Input: part model. Units: mm. Frame: model coordinates. A direction names the side the tool comes from. Give positions to 0.01 mm unless a question says otherwise; leave off trailing zeros. Order: outer loops, then holes, each group sorted by start corner. A loop starts at its lowest first (then second) coordinate and runs counter-clockwise, first axis right, second up. Notation, with made-up numbers: (17.25, -19) - (39.25, -19) arc R23 ccw to (39.25, 5) - close; hole circle Ø4 at (81.5, 10.5). An arc over 180 degrees is marked (long way). Answer in a Markdown table with one row per item. Add a question column.
1. Section query B-B on x = 50. Return loops of the section in (y, z) (1 decimal), and give its area (3 significant figures).
2. Access query for faces 5 (the face through (-4, 50.8, -23)), 6 (the face through (280.988, 3, -15)). Directions: +Z, -Z, +X, -X, +Y, -Y. A direction counts if a zero-diameter tool reaches every point of the face in a straight line with its end or side. Return the directions, or none.
3. Ray query, line 1 (Y direction, x = 109.5, z = 36) (3 decimals); line 2 (Y direction, x = -187.5, z = -9.5) (3 decimals); line 3 (Z direction, x = 96, y = 49.5). Return the intervals inside material, ascending. Write a range as [from, to].
4. Section query C-C on z = 41. Return loops of the section in (x, y) (1 decimal), and give its area (3 significant figures).
5. Section query D-D on y = 15. Return loops of the section in (x, z), and give its area (3 significant figures).
6. Mould query, pull axis Y, two halves, no side actions, for faces 1 (the face through (5, 3.175, 2)), 2 (the face through (4, 0, 1)), 3 (the face through (-277.812, 29, 2)), 4 (the face through (217.632, 52.41, 5.074)). Classes: released by +Y, released by -Y, zero draft, split by the parting line, or undercut.
7. Contact query for flat-ended pins moving along their axis: pin 1 (2 mm diameter, centred on y = 10, z = 14, fed in from +X); pin 2 (3.5 mm diameter, centred on y = 52, z = -0.5, fed in from +X); pin 3 (8 mm diameter, centred on x = -93, y = 13.5, fed in from +Z). Output: stop coordinate, or through.
8. Section query A-A on z = -32. Return loops of the section in (x, y) (1 decimal), and give its area (3 significant figures).
Autodesk Inventor part; units mm, degrees
ref_plane "YZ Plane" through (0, 0, 0) normal (1, 0, 0) x (0, 1, 0)
ref_plane "XZ Plane" through (0, 0, 0) normal (0, 1, 0) x (-1, 0, 0)
ref_plane "XY Plane" through (0, 0, 0) normal (0, 0, 1) x (1, 0, 0)
sketch "Sketch1" plane through (0, 0, 0) normal (0, 1, 0) x (-1, 0, 0)
  line L0 (-280.9875, -52.3875) -> (-280.9875, 52.3875)
  line L1 (-280.9875, 52.3875) -> (280.9875, 52.3875)
  line L2 (280.9875, 52.3875) -> (280.9875, -52.3875)
  line L3 (280.9875, -52.3875) -> (-280.9875, -52.3875)
  line L4 (-280.9875, -52.3875) -> (280.9875, 52.3875) construction
  line L5 (-280.9875, 52.3875) -> (280.9875, -52.3875) construction
  line L6 (0, -52.3875) -> (0, -17.4625) construction
  line L7 (-277.8125, -49.2125) -> (277.8125, -49.2125)
  line L8 (277.8125, -49.2125) -> (277.8125, 49.2125)
  line L9 (277.8125, 49.2125) -> (-277.8125, 49.2125) construction
  line L10 (-277.8125, 49.2125) -> (-277.8125, -49.2125)
  line L11 (-277.8125, -49.2125) -> (277.8125, 49.2125) construction
  line L12 (277.8125, -49.2125) -> (-277.8125, 49.2125) construction
  line L13 (277.8125, 49.2125) -> (277.8125, 52.3875)
  line L14 (-277.8125, 49.2125) -> (-277.8125, 52.3875)
  point P0 (0, 0)
  dimension "d0" = 104.775
  dimension "d1" = 561.975
  dimension "d2" = 34.925
  dimension "d3" = 555.625
  dimension "d4" = 98.425
extrude "Extrusion1" add sketch "Sketch1" along normal blind 3.175 contours L1 L13 L8 L7 L10 L14
extrude "Extrusion2" add sketch "Sketch1" along normal blind 50.8 contours L0 L1 L14 L10 L7 L8 L13 L2 L3
sketch "Sketch2" plane through (0, 50.8, 0) normal (0, 1, 0) x (1, 0, 0)
  line L0 (-280.9875, -52.3875) -> (-277.8125, -52.3875)
  line L1 (-280.9875, -52.3875) -> (255.5875, -52.3875)
  line L2 (280.9875, -52.3875) -> (280.9875, -26.9875)
  line L3 (-280.9875, -26.9875) -> (-280.9875, -52.3875)
  line L4 (-280.9875, 52.3875) -> (-280.9875, -52.3875)
  line L5 (-280.9875, 52.3875) -> (255.5875, 52.3875)
  line L6 (280.9875, 52.3875) -> (280.9875, 17.4625)
  line L7 (-280.9875, 17.4625) -> (-280.9875, 52.3875)
  line L8 (-280.9875, 52.3875) -> (-255.5875, 52.3875)
  line L9 (-255.5875, -52.3875) -> (-280.9875, -52.3875)
  line L10 (-280.9875, -52.3875) -> (-280.9875, -26.9875)
  line L11 (-277.8125, -52.3875) -> (277.8125, -52.3875)
  line L12 (280.9875, 52.3875) -> (255.5875, 52.3875)
  line L13 (255.5875, -52.3875) -> (280.9875, -52.3875)
  line L14 (280.9875, -52.3875) -> (280.9875, 17.4625)
  line L15 (255.5875, 17.4625) -> (255.5875, -26.9875)
  line L16 (255.5875, 17.4625) -> (-255.5875, 17.4625)
  line L17 (255.5875, 52.3875) -> (280.9875, 52.3875)
  line L18 (280.9875, 17.4625) -> (280.9875, 52.3875)
  line L19 (255.5875, -26.9875) -> (-255.5875, -26.9875)
  line L20 (255.5875, -52.3875) -> (280.9875, -52.3875)
  line L21 (-255.5875, 17.4625) -> (-255.5875, -26.9875)
  line L22 (-280.9875, 17.4625) -> (-280.9875, 52.3875)
  line L23 (-280.9875, -26.9875) -> (-280.9875, 17.4625)
  line L24 (-277.8125, -52.3875) -> (-277.8125, 49.2125) construction
  line L25 (-277.8125, -52.3875) -> (-277.8125, -49.2125) construction
  line L26 (-277.8125, -49.2125) -> (277.8125, -49.2125)
  line L27 (-277.8125, -49.2125) -> (-277.8125, -52.3875)
  line L28 (277.8125, -49.2125) -> (277.8125, -52.3875)
  point P0 (0, 0)
  dimension "d9" = 561.975
  dimension "d10" = 25.4
  dimension "d11" = 561.975
  dimension "d12" = 34.925
  dimension "d13" = 25.4
  dimension "d14" = 104.775
  dimension "d15" = 25.4
  dimension "d18" = 3.175
  dimension "d19" = 555.625
extrude "Extrusion3" add sketch "Sketch2" along normal blind 3.175
sketch "Sketch3" plane through (0, 53.975, 0) normal (0, 1, 0) x (1, 0, 0)
  line L0 (-277.8125, -52.3875) -> (-277.8125, 49.2125)
  line L1 (-277.8125, -52.3875) -> (277.8125, -52.3875)
  line L2 (277.8125, -52.3875) -> (277.8125, -49.2125)
  line L3 (277.8125, -49.2125) -> (-277.8125, -49.2125)
  line L4 (-277.8125, -49.2125) -> (-277.8125, -52.3875)
  point P0 (0, 0)
  dimension "d20" = 555.625
  dimension "d21" = 3.175
extrude "Extrusion4" cut sketch "Sketch3" against normal blind 3.175
sketch "Sketch4" plane through (280.9875, 0, 52.3875) normal (1, 0, 0) x (0, 0, -1)
  line L0 (3.175, 53.975) -> (0, 53.975)
  line L1 (0, 53.975) -> (104.775, 53.975)
  line L2 (104.775, 53.975) -> (104.775, 0)
  line L3 (0, 0) -> (0, 53.975)
  line L4 (52.3875, 0) -> (52.3875, 3.175) construction
  line L5 (0, 3.175) -> (101.6, 3.175) construction
  line L6 (0, 3.175) -> (104.775, 3.175)
  line L7 (104.775, 0) -> (104.775, 53.975)
extrude "Extrusion5" cut sketch "Sketch4" against normal blind 3.175
sketch "Sketch5" plane through (0, 53.975, 0) normal (0, 1, 0) x (1, 0, 0)
  line L0 (255.5875, -26.9875) -> (255.5875, 17.4625)
  line L1 (255.5875, -26.9875) -> (178.5978, 17.4625)
  line L2 (255.5875, 17.4625) -> (-255.5875, 17.4625)
  line L3 (255.5875, -26.9875) -> (344.4875, -26.9875) construction
  line L4 (178.5978, 17.4625) -> (255.5875, 17.4625)
  point P0 (0, 0)
  dimension "d26" = 150
extrude "Extrusion6" add sketch "Sketch5" against normal blind 3.175
sketch "Sketch6" plane through (277.8125, 0, 52.3875) normal (1, 0, 0) x (0, 0, -1)
  line L0 (104.775, 0) -> (104.775, 53.975)
  line L1 (104.775, 50.8) -> (104.775, 53.975)
  line L2 (104.775, 53.975) -> (101.6, 53.975)
  line L3 (101.6, 3.175) -> (104.775, 3.175)
  line L4 (104.775, 3.175) -> (104.775, 50.8)
  line L5 (101.6, 50.8) -> (101.6, 3.175)
  line L6 (101.6, 50.8) -> (101.6, 53.975)
  point P0 (52.3875, 0)
  point P1 (3.175, 50.8)
extrude "Extrusion7" add sketch "Sketch6" along normal blind 3.175
sketch "Sketch8" plane through (0, 3.175, 0) normal (0, 1, 0) x (1, 0, 0)
  line L0 (277.8125, -49.2125) -> (277.8125, 49.2125)
  line L1 (277.8125, 49.2125) -> (279.4635, 49.2125)
  line L2 (279.4635, 49.2125) -> (279.4635, 23.6855)
  line L3 (279.4635, 23.6855) -> (277.8125, 23.6855)
  line L4 (277.8125, 23.6855) -> (277.8125, 49.2125)
  point P0 (0, 0)
  dimension "d36" = 1.651
  dimension "d37" = 25.527
extrude "Extrusion9" cut sketch "Sketch8" against normal blind 3.175
properties part number "Wire Housing No Support Struct vglue"
Answer:
| question | item | result |
|---|---|---|
| 1 | outline | (0, -52.4) - (54, -52.4) - (54, -17.5) - (50.8, -17.5) - (50.8, -49.2) - (3.2, -49.2) - (3.2, 52.4) - (0, 52.4) - close; (50.8, 27) - (54, 27) - (54, 49.2) - (50.8, 49.2) - close |
| 1 | area | 665 mm² |
| 2 | face 5 | +Z, +X |
| 2 | face 6 | +Z, -Z, +X, +Y, -Y |
| 3 | line 1 | y = [0, 3.175], [50.8, 53.975] |
| 3 | line 2 | y = [0, 3.175] |
| 3 | line 3 | z = [-52.39, -49.21] |
| 4 | outline | (-281, 0) - (281, 0) - (281, 3.2) - (-277.8, 3.2) - (-277.8, 50.8) - (277.8, 50.8) - (277.8, 54) - (-281, 54) - close |
| 4 | area | 3,710 mm² |
| 5 | outline | (-280.99, -52.39) - (280.99, -52.39) - (280.99, -49.21) - (-277.81, -49.21) - (-277.81, 52.39) - (-280.99, 52.39) - close |
| 5 | area | 2,110 mm² |
| 6 | face 1 | undercut |
| 6 | face 2 | released by -Y |
| 6 | face 3 | undercut |
| 6 | face 4 | zero draft |
| 7 | pin 1 | stops at x = -277.81 |
| 7 | pin 2 | stops at x = 277.81 |
| 7 | pin 3 | stops at z = -49.21 |
| 8 | outline | (-281, 0) - (277.8, 0) - (277.8, 3.2) - (-277.8, 3.2) - (-277.8, 50.8) - (277.8, 50.8) - (277.8, 54) - (-281, 54) - close; (279.5, 0) - (281, 0) - (281, 3.2) - (279.5, 3.2) - close |
| 8 | area | 3,700 mm² |
